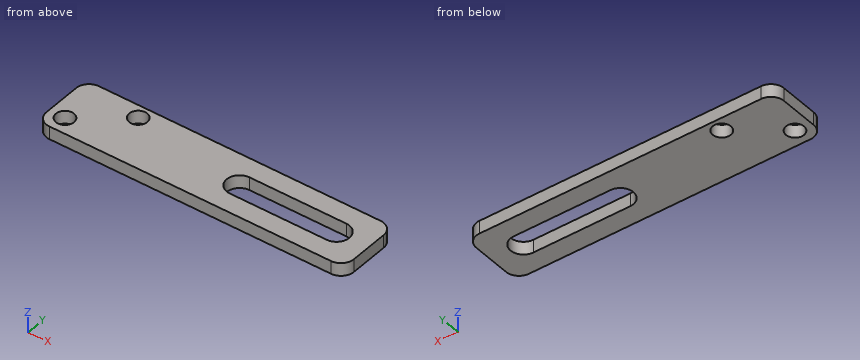
```python
from build123d import *

# Parameters (mm, degrees)
F0_R     = 1.4
F1_DEPTH = 2
F2_R     = 2
F4_DEPTH = 2.001


with BuildPart() as f1:
    # F0 (on Top) → F1 (new body)
    with BuildSketch(Plane.XY):
        Polygon((47.623903, 0), (47.623903, 10), (13.023903, 10), (0, 10), (0, 0), align=None)
        with Locations((2.5, 2.5)):
            Circle(F0_R, mode=Mode.SUBTRACT)
        with Locations((9.623903, 8)):
            Circle(F0_R, mode=Mode.SUBTRACT)
    extrude(amount=F1_DEPTH)

    # F2
    f2_edges = [f1.edges().sort_by_distance(p)[0] for p in [
        (0, 0, 1),
        (0, 10, 1),
        (47.623903, 0, 1),
        (47.623903, 10, 1),
    ]]
    fillet(f2_edges, radius=F2_R)

    # F3 (on face) → F4 (cut, through all)
    with BuildSketch(Plane.XY.offset(2)):
        with BuildLine():
            ThreePointArc((42.623903, 3), (44.623903, 5), (42.623903, 7))
            Line((42.623903, 7), (27.623903, 7))
            ThreePointArc((27.623903, 7), (25.623903, 5), (27.623903, 3))
            Line((27.623903, 3), (42.623903, 3))
        make_face()
    extrude(amount=-F4_DEPTH, mode=Mode.SUBTRACT)


solid = f1.part
```
Work out the finished part from the listing and answer in its coordinate system (mm). Round coordinates to 2 decimals unless told otherwise and drop trailing zeros. Write each loop counter-clockwise with the first axis right and the second up, starting at its lowest first coordinate (ties: lowest second). Pieces come first, ordered by that corner, then holes.
1) A cutting plane is placed at B-B on y = 5. Determine the outline of the cut face in (x, z), and give its area (3 significant figures).
2) Consider probe 1 along Y at (x, z) = (35, 1.95); probe 2 along Y at (x, z) = (2.5, 0.85); probe 3 along X at (y, z) = (5.25, 0.5). Determine where each line is inside the solid, lowest interval first.
3) A cutting plane is placed at A-A on x = 2.5. Determine the outline of the cut face in (y, z), and give its area (3 significant figures).
4) A cutting plane is placed at C-C on z = 0.8. Determine the outline of the cut face in (x, y).
Entries:
1. outline: (0, 0) - (25.62, 0) - (25.62, 2) - (0, 2) - close; (44.62, 0) - (47.62, 0) - (47.62, 2) - (44.62, 2) - close
1. area: 57.2 mm2
2. probe 1: y = 0 to 3, 7 to 10
2. probe 2: y = 0 to 1.1, 3.9 to 10
2. probe 3: x = 0 to 25.64, 44.61 to 47.62
3. outline: (0, 0) - (1.1, 0) - (1.1, 2) - (0, 2) - close; (3.9, 0) - (10, 0) - (10, 2) - (3.9, 2) - close
3. area: 14.4 mm2
4. outline: (0, 2) arc R2 ccw to (2, 0) - (45.62, 0) arc R2 ccw to (47.62, 2) - (47.62, 8) arc R2 ccw to (45.62, 10) - (2, 10) arc R2 ccw to (0, 8) - close; hole circle Ø2.8 at (2.5, 2.5); hole circle Ø2.8 at (9.62, 8); hole (27.62, 3) - (42.62, 3) arc R2 ccw to (42.62, 7) - (27.62, 7) arc R2 ccw to start
